Geometry: final body of the model. Coordinates: model frame, mm. Round coordinates to 2 decimals unless told otherwise and drop trailing zeros. Loops run counter-clockwise (first coordinate to the right, second up) from the corner with the lowest first, then second, coordinate; pieces in that order, holes last. Notation, with made-up numbers: (28.25, 47.25) - (55.25, 47.25) arc R30 ccw to (55.25, 70.25) - close; hole circle Ø10 at (71.25, -4). An arc over 180 degrees is marked (long way). Answer as CSV lines item,"result".
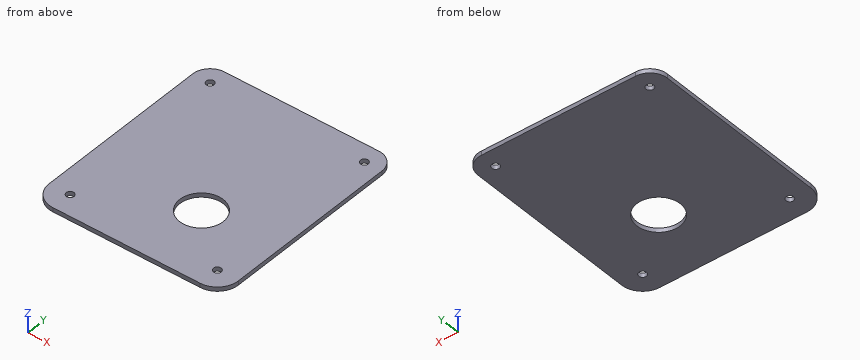
from build123d import *

# Parameters (mm, degrees)
BASE_FLANGE1_DEPTH   = 3
SKETCH2_R            = 15.5
CUT_EXTRUDE1_DEPTH   = 131.05864062
M5_CLEARANCE_HOLE1_D = 5.5


# Sheet-metal steps are written as plain solids
with BuildPart() as part:
    # Sketch1 → Base-Flange1 (new body)
    with BuildSketch(Plane.XY):
        with BuildLine():
            Line((-67.5, 102.5), (42.5, 102.5))
            ThreePointArc((42.5, 102.5), (51.338834765, 98.838834765), (55, 90))
            Line((55, 90), (55, -35))
            ThreePointArc((55, -35), (50.606601718, -45.606601718), (40, -50))
            Line((40, -50), (-65, -50))
            ThreePointArc((-65, -50), (-75.606601718, -45.606601718), (-80, -35))
            Line((-80, -35), (-80, 90))
            ThreePointArc((-80, 90), (-76.338834765, 98.838834765), (-67.5, 102.5))
        make_face()
    extrude(amount=BASE_FLANGE1_DEPTH)

    # Sketch2 → Cut-Extrude1 (cut, through all)
    with BuildSketch(Plane.XY.offset(3)):
        Circle(SKETCH2_R)
    extrude(amount=-CUT_EXTRUDE1_DEPTH, mode=Mode.SUBTRACT)

    # M5 Clearance Hole1 (through all)
    with Locations(Plane(origin=(0, 0, 0), x_dir=(-1, 0, 0), z_dir=(0, 0, -1))):
        with Locations((-40, -35), (67.5, 90), (65, -35), (-42.5, 90)):
            Hole(M5_CLEARANCE_HOLE1_D / 2)


solid = part.part
(1) Section B-B (y = 0). Output: boundary loops of the cut face in (x, z).
Findings below:
outline,"(-80, 0) - (-15.5, 0) - (-15.5, 3) - (-80, 3) - close; (15.5, 0) - (55, 0) - (55, 3) - (15.5, 3) - close"
(2) Section C-C (x = 2.5). Output: boundary loops of the cut face in (y, z).
Findings below:
outline,"(-50, 0) - (-15.3, 0) - (-15.3, 3) - (-50, 3) - close; (15.3, 0) - (102.5, 0) - (102.5, 3) - (15.3, 3) - close"
(3) Material intervals for line 1 along Y through (x, z) = (0, 0.95); line 2 along Y through (x, z) = (-67.5, 1); line 3 along X through (y, z) = (89, 1.7), sorted ascending.
Findings below:
line 1,"-50 to -15.5, 15.5 to 102.5"
line 2,"-49.79 to -36.15, -33.85 to 87.25, 92.75 to 102.5"
line 3,"-80 to -70.06, -64.94 to 39.94, 45.06 to 55"
(4) Section A-A (z = 2.05). Output: boundary loops of the cut face in (x, y), and give its area (3 significant figures).
Findings below:
outline,"(-80, -35) arc R15 ccw to (-65, -50) - (40, -50) arc R15 ccw to (55, -35) - (55, 90) arc R12.5 ccw to (42.5, 102.5) - (-67.5, 102.5) arc R12.5 ccw to (-80, 90) - close; hole circle Ø5.5 at (-67.5, 90); hole circle Ø5.5 at (-65, -35); hole circle Ø31 at (0, 0); hole circle Ø5.5 at (40, -35); hole circle Ø5.5 at (42.5, 90)"
area,"19,600 mm2"
